Work out the finished part from the listing and answer in its coordinate system (mm). Face numbers are marked on the shaded views. A direction names the side the tool comes from. Round coordinates to 2 decimals unless told otherwise and drop trailing zeros. Write each loop counter-clockwise with the first axis right and the second up, starting at its lowest first coordinate (ties: lowest second). Pieces come first, ordered by that corner, then holes. Notation, with made-up numbers: (-12, 40.25) - (26, 40.25) arc R26 cw to (26, 73.25) - close; hole circle Ø1 at (49, -30.5). An arc over 180 degrees is marked (long way). Write item = value, one per line. Start each with the question number.
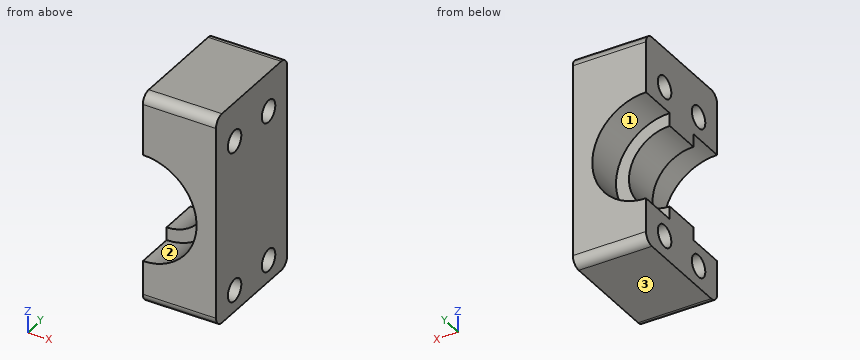
from build123d import *

# Parameters (mm, degrees)
SKETCH8_W           = 30
SKETCH8_H           = 100
BOSS_EXTRUDE1_DEPTH = 100
SKETCH9_W           = 88.7
SKETCH9_H           = 30
CUT_EXTRUDE1_DEPTH  = 103.708324882
SKETCH10_R          = 1.7
CUT_EXTRUDE2_DEPTH  = 21.825225089
MOVE_FACE1_BY       = 2.7
FILLET1_R           = 1.5


with BuildPart() as part:
    # Sketch8 → Boss-Extrude1 (new body)
    with BuildSketch(Plane(origin=(0, 0, 0), x_dir=(0, 0, -1), z_dir=(1, 0, 0))):
        Rectangle(SKETCH8_W, SKETCH8_H)
    extrude(amount=BOSS_EXTRUDE1_DEPTH)

    # Sketch7 → Cut-Revolve3 (revolve, cut)
    with BuildSketch(Plane(origin=(0, 0, 0), x_dir=(0, 0, -1), z_dir=(1, 0, 0))):
        Polygon((-8.3, 9), (-150, 9), (-150, 50), (0, 50), (0, -50), (-150, -50), (-150, -9), (-8.3, -9), (-8.3, -3), (-6.3, -3), (-6.3, 3), (-8.3, 3), align=None)
    revolve(axis=Axis((0, -50, 0), (0, 1, 0)), mode=Mode.SUBTRACT)

    # Sketch9 → Cut-Extrude1 (cut, through all)
    with BuildSketch(Plane(origin=(0, 9, 0), x_dir=(1, 0, 0), z_dir=(0, 1, 0))):
        with Locations((55.65, 0)):
            Rectangle(SKETCH9_W, SKETCH9_H)
    extrude(amount=-CUT_EXTRUDE1_DEPTH, mode=Mode.SUBTRACT)

    # Sketch10 → Cut-Extrude2 (cut, through all)
    with BuildSketch(Plane.ZY):
        with Locations((-11.65, 4.3)):
            Circle(SKETCH10_R)
        with Locations((-11.65, -4.3)):
            Circle(SKETCH10_R)
        with Locations((11.65, -4.3)):
            Circle(SKETCH10_R)
        with Locations((11.65, 4.3)):
            Circle(SKETCH10_R)
    extrude(amount=-CUT_EXTRUDE2_DEPTH, mode=Mode.SUBTRACT)

    # Move Face1: a face moved outward by 2.7
    extrude(part.faces().sort_by_distance((5.65, 0, 15))[0], amount=MOVE_FACE1_BY, dir=(0, 0, 1))

    # Fillet1
    fillet1_edges = [part.edges().sort_by_distance(p)[0] for p in [
        (5.65, 9, 17.7),
        (5.65, -9, -15),
        (5.65, -9, 17.7),
        (5.65, 9, -15),
    ]]
    fillet(fillet1_edges, radius=FILLET1_R)


solid = part.part
1. Each of these flat-tipped pins is pushed along its axis until it touches: pin 1 (2.5 mm diameter, centred on y = 4.3, z = 11.65, fed in from +X); pin 2 (4.5 mm diameter, centred on y = -4.3, z = 11.65, fed in from -X); pin 3 (4 mm diameter, centred on x = 5.5, z = 2.5, fed in from +Y). Where does it stop, or does it pass through?
2. Find section C-C on z = 11.65. Give the vertices of the cut face in (x, y).
3. Find section B-B on y = 4.3. Give the vertices of the cut face in (x, z).
4. Which of the six approach directions +Z, -Z, +X, -X, +Y, -Y give full straight-line access (tool end or side, diameter ignored) to the marked faces 1, 2 and 3?
5. Consider line 1 (Y direction, x = 2.5, z = 11.65); line 2 (Y direction, x = 3.25, z = -12.5); line 3 (Z direction, x = 6.5, y = -2.75). Determine where each line is inside the solid, lowest interval first.
6. Find section D-D on x = 9.25. Give the vertices of the cut face in (y, z).
7. Find section A-A on x = 3.5. Give the vertices of the cut face in (y, z).
Answer key:
q1.pin_1 = through
q1.pin_2 = 0
q1.pin_3 = 3
q2.outline = (0, -9) - (11.3, -9) - (11.3, -6) - (0, -6) - close; (0, -2.6) - (11.3, -2.6) - (11.3, 2.6) - (0, 2.6) - close; (0, 6) - (11.3, 6) - (11.3, 9) - (0, 9) - close
q3.outline = (0, -15) - (11.3, -15) - (11.3, -13.35) - (0, -13.35) - close; (0, -9.95) - (11.3, -9.95) - (11.3, 9.95) - (0, 9.95) - (0, 8.3) arc R8.3 cw to (0, -8.3) - close; (0, 13.35) - (11.3, 13.35) - (11.3, 17.7) - (0, 17.7) - close
q4.face_1 = -X, +Y
q4.face_2 = -X, -Y
q4.face_3 = -Z, +X, -X, +Y, -Y
q5.line_1 = -9 to -6, -2.6 to 2.6, 6 to 9
q5.line_2 = -9 to -5.77, -2.83 to 2.83, 5.77 to 9
q5.line_3 = -15 to -12.35, -10.95 to 10.95, 12.35 to 17.7
q6.outline = (-9, -13.5) arc R1.5 ccw to (-7.5, -15) - (7.5, -15) arc R1.5 ccw to (9, -13.5) - (9, 16.2) arc R1.5 ccw to (7.5, 17.7) - (-7.5, 17.7) arc R1.5 ccw to (-9, 16.2) - close; hole circle Ø3.4 at (-4.3, -11.65); hole circle Ø3.4 at (-4.3, 11.65); hole circle Ø3.4 at (4.3, -11.65); hole circle Ø3.4 at (4.3, 11.65)
q7.outline = (-9, -13.5) arc R1.5 ccw to (-7.5, -15) - (7.5, -15) arc R1.5 ccw to (9, -13.5) - (9, -7.53) - (3, -7.53) - (3, -5.24) - (-3, -5.24) - (-3, -7.53) - (-9, -7.53) - close; (-9, 7.53) - (-3, 7.53) - (-3, 5.24) - (3, 5.24) - (3, 7.53) - (9, 7.53) - (9, 16.2) arc R1.5 ccw to (7.5, 17.7) - (-7.5, 17.7) arc R1.5 ccw to (-9, 16.2) - close; hole circle Ø3.4 at (-4.3, -11.65); hole circle Ø3.4 at (-4.3, 11.65); hole circle Ø3.4 at (4.3, -11.65); hole circle Ø3.4 at (4.3, 11.65)
